Here's how the part is built. I have some questions about the finished solid (model axes, mm). Face numbers are marked on the shaded views. A direction names the side the tool comes from. Coordinates: 2 decimals unless noted, no trailing zeros. Write each loop counter-clockwise with the first axis right and the second up, starting at its lowest first coordinate (ties: lowest second). Pieces come first, ordered by that corner, then holes.
Item 1: I'm going to push flat-ended pins straight in: pin 1 Ø2 at (x, y) = (42.5, -18.5) entering from +Z (3 decimals); pin 2 Ø12 at (y, z) = (-23.5, 36) entering from +X; pin 3 Ø2 at (y, z) = (-110, 72.5) entering from +X. Where does each tip first touch, or does it pass through?
Item 2: If we section it at B-B (x = 30): Please give me the cut outline in (y, z) (3 decimals), then the cut area to 3 significant figures.
Item 3: We'd pull the mould along Z, two halves only. Please class the marked faces 1, 2 and 3: +Z half, -Z half, draft (parallel to the pull), parting line (faces both ways), or undercut.
Item 4: If we section it at A-A (z = 46): Please give me the cut outline in (x, y), then the cut area to 3 significant figures.
Item 5: For the marked faces 4 and 5, which set-ups out of +Z, -Z, +X, -X, +Y, -Y let a thin tool reach every point of the face, with its end or its side?
Item 6: If I drill on line 1 (Z direction, x = 29.5, y = -147) (3 decimals); line 2 (Z direction, x = 107.5, y = 131.5) (3 decimals); line 3 (Y direction, x = 68.5, z = 47), over which ranges is the centre line in solid material (lowest first)?
Item 7: If we section it at D-D (x = 147): Please give me the cut outline in (y, z) (3 decimals), then the cut area to 3 significant figures.
from build123d import *

# Parameters (mm, degrees)
F1_DEPTH = 3.175
F3_DEPTH = 76.2
F5_DEPTH = 3.175


with BuildPart() as f1:
    # F0 (on Top) → F1 (new body)
    with BuildSketch(Plane.XY):
        with BuildLine():
            ThreePointArc((0, 152.4), (23.5583821583, 150.5681328505), (46.5504148891, 145.1165699486))
            Line((46.5504148891, 145.1165699486), (76.2, 145.1165699486))
            Line((76.2, 145.1165699486), (76.2, 220.9699887776))
            Line((76.2, 220.9699887776), (0, 220.9699887776))
            Line((0, 220.9699887776), (0, 152.4))
        make_face()
        with BuildLine():
            Line((0, 145.1165699486), (46.5504148891, 145.1165699486))
            ThreePointArc((46.5504148891, 145.1165699486), (23.5583821583, 150.5681328505), (0, 152.4))
            Line((0, 152.4), (0, 145.1165699486))
        make_face()
        with BuildLine():
            Line((76.2, 79.9558987255), (76.2, 131.9822715367))
            ThreePointArc((76.2, 131.9822715367), (61.7255501195, 139.3402901621), (46.5504148891, 145.1165699486))
            Line((46.5504148891, 145.1165699486), (0, 145.1165699486))
            Line((0, 145.1165699486), (0, 102.5676841179))
            ThreePointArc((0, 102.5676841179), (39.7420836099, 96.795488514), (76.2, 79.9558987255))
        make_face()
        with BuildLine():
            Line((76.2, 30.069767419), (76.2, 79.9558987255))
            ThreePointArc((76.2, 79.9558987255), (39.7420836099, 96.795488514), (0, 102.5676841179))
            Line((0, 102.5676841179), (0, 64.4676841179))
            ThreePointArc((0, 64.4676841179), (41.802083301, 55.469767419), (76.2, 30.069767419))
        make_face()
        with BuildLine():
            ThreePointArc((134.4041666021, 0.9676841179), (112.4647200648, 45.7397345375), (76.2, 79.9558987255))
            Line((76.2, 79.9558987255), (76.2, 30.069767419))
            ThreePointArc((76.2, 30.069767419), (86.426594721, 16.2812004311), (94.1857207861, 0.9676841179))
            Line((94.1857207861, 0.9676841179), (134.4041666021, 0.9676841179))
        make_face()
        with BuildLine():
            ThreePointArc((94.1857207861, 0.9676841179), (86.426594721, 16.2812004311), (76.2, 30.069767419))
            Line((76.2, 30.069767419), (76.2, 0.9676841179))
            Line((76.2, 0.9676841179), (94.1857207861, 0.9676841179))
        make_face()
        with BuildLine():
            Line((94.1857207861, 0.9676841179), (76.2, 0.9676841179))
            Line((76.2, 0.9676841179), (76.2, -104.3343991831))
            ThreePointArc((76.2, -104.3343991831), (95.0380976241, -73.0533403663), (101.6, -37.1323158821))
            ThreePointArc((101.6, -37.1323158821), (99.7292064339, -17.7249620165), (94.1857207861, 0.9676841179))
        make_face()
        with BuildLine():
            ThreePointArc((0, -152.4), (39.4440224736, -147.2070959265), (76.2, -131.9822715367))
            Line((76.2, -131.9822715367), (76.2, -104.3343991831))
            ThreePointArc((76.2, -104.3343991831), (41.802083301, -129.7343991831), (0, -138.7323158821))
            Line((0, -138.7323158821), (0, -152.4))
        make_face()
        with BuildLine():
            Line((76.2, -104.3343991831), (76.2, 0.9676841179))
            Line((76.2, 0.9676841179), (0, 0.9676841179))
            Line((0, 0.9676841179), (0, -138.7323158821))
            ThreePointArc((0, -138.7323158821), (41.802083301, -129.7343991831), (76.2, -104.3343991831))
        make_face()
        with BuildLine():
            Line((76.2, -154.2205304897), (76.2, -131.9822715367))
            ThreePointArc((76.2, -131.9822715367), (39.4440224736, -147.2070959265), (0, -152.4))
            Line((0, -152.4), (0, -166.4440847683))
            Line((0, -166.4440847683), (52.8635642719, -166.4440847683))
            ThreePointArc((52.8635642719, -166.4440847683), (64.8205578921, -160.8836200148), (76.2, -154.2205304897))
        make_face()
        with BuildLine():
            Line((0, -236.2300112224), (76.2, -236.2300112224))
            Line((76.2, -236.2300112224), (76.2, -166.4440847683))
            Line((76.2, -166.4440847683), (52.8635642719, -166.4440847683))
            ThreePointArc((52.8635642719, -166.4440847683), (26.9372965106, -174.2106586525), (0, -176.8323158821))
            Line((0, -176.8323158821), (0, -236.2300112224))
        make_face()
        Polygon((76.2, -236.2300112224), (101.6, -166.4440847683), (76.2, -166.4440847683), align=None)
        with BuildLine():
            Line((76.2, -166.4440847683), (76.2, -154.2205304897))
            ThreePointArc((76.2, -154.2205304897), (64.8205578921, -160.8836200148), (52.8635642719, -166.4440847683))
            Line((52.8635642719, -166.4440847683), (76.2, -166.4440847683))
        make_face()
        with BuildLine():
            ThreePointArc((0, -176.8323158821), (26.9372965106, -174.2106586525), (52.8635642719, -166.4440847683))
            Line((52.8635642719, -166.4440847683), (0, -166.4440847683))
            Line((0, -166.4440847683), (0, -176.8323158821))
        make_face()
        with BuildLine():
            Line((101.6, -166.4440847683), (131.2750589092, -84.9125304942))
            ThreePointArc((131.2750589092, -84.9125304942), (109.372641612, -124.0444281957), (76.2, -154.2205304897))
            Line((76.2, -154.2205304897), (76.2, -166.4440847683))
            Line((76.2, -166.4440847683), (101.6, -166.4440847683))
        make_face()
        with BuildLine():
            ThreePointArc((131.2750589092, -84.9125304942), (133.9529126579, -76.7896883426), (136.1286754731, -68.5181998738))
            ThreePointArc((136.1286754731, -68.5181998738), (110.8051835658, -104.6325537056), (76.2, -131.9822715367))
            Line((76.2, -131.9822715367), (76.2, -154.2205304897))
            ThreePointArc((76.2, -154.2205304897), (109.372641612, -124.0444281957), (131.2750589092, -84.9125304942))
        make_face()
        with BuildLine():
            ThreePointArc((76.2, -131.9822715367), (110.8051835658, -104.6325537056), (136.1286754731, -68.5181998738))
            ThreePointArc((136.1286754731, -68.5181998738), (138.8042974183, -52.9265242574), (139.7, -37.1323158821))
            ThreePointArc((139.7, -37.1323158821), (138.3697078018, -17.8991683798), (134.4041666021, 0.9676841179))
            Line((134.4041666021, 0.9676841179), (94.1857207861, 0.9676841179))
            ThreePointArc((94.1857207861, 0.9676841179), (99.7292064339, -17.7249620165), (101.6, -37.1323158821))
            ThreePointArc((101.6, -37.1323158821), (95.0380976241, -73.0533403663), (76.2, -104.3343991831))
            Line((76.2, -104.3343991831), (76.2, -131.9822715367))
        make_face()
        with BuildLine():
            ThreePointArc((143.2091555839, -52.1238693589), (150.0847016038, -26.4639820229), (152.4, 0))
            ThreePointArc((152.4, 0), (131.9822715367, 76.2), (76.2, 131.9822715367))
            Line((76.2, 131.9822715367), (76.2, 79.9558987255))
            ThreePointArc((76.2, 79.9558987255), (112.4647200648, 45.7397345375), (134.4041666021, 0.9676841179))
            ThreePointArc((134.4041666021, 0.9676841179), (138.3697078018, -17.8991683798), (139.7, -37.1323158821))
            ThreePointArc((139.7, -37.1323158821), (138.8042974183, -52.9265242574), (136.1286754731, -68.5181998738))
            ThreePointArc((136.1286754731, -68.5181998738), (139.9092544586, -60.4248336103), (143.2091555839, -52.1238693589))
        make_face()
        with BuildLine():
            ThreePointArc((76.2, 131.9822715367), (131.9822715367, 76.2), (152.4, 0))
            ThreePointArc((152.4, 0), (150.0847016038, -26.4639820229), (143.2091555839, -52.1238693589))
            Line((143.2091555839, -52.1238693589), (242.6071911065, 220.9699887776))
            Line((242.6071911065, 220.9699887776), (76.2, 145.1165699486))
            Line((76.2, 145.1165699486), (76.2, 131.9822715367))
        make_face()
        with BuildLine():
            ThreePointArc((46.5504148891, 145.1165699486), (61.7255501195, 139.3402901621), (76.2, 131.9822715367))
            Line((76.2, 131.9822715367), (76.2, 145.1165699486))
            Line((76.2, 145.1165699486), (46.5504148891, 145.1165699486))
        make_face()
        Polygon((76.2, 220.9699887776), (76.2, 145.1165699486), (242.6071911065, 220.9699887776), align=None)
        with BuildLine():
            Line((131.2750589092, -84.9125304942), (143.2091555839, -52.1238693589))
            ThreePointArc((143.2091555839, -52.1238693589), (139.9092544586, -60.4248336103), (136.1286754731, -68.5181998738))
            ThreePointArc((136.1286754731, -68.5181998738), (133.9529126579, -76.7896883426), (131.2750589092, -84.9125304942))
        make_face()
    extrude(amount=F1_DEPTH)

    # F2 (on face) → F3 (join)
    with BuildSketch(Plane.XY.offset(3.175)):
        Polygon((242.6071911065, 220.9699887776), (239.2284266789, 220.9699887776), (73.9768410662, -233.0550112224), (77.3556054938, -233.0550112224), align=None)
        Polygon((77.3556054938, -233.0550112224), (73.9768410662, -233.0550112224), (72.8212355724, -236.2300112224), (76.2, -236.2300112224), align=None)
        Polygon((72.8212355724, -236.2300112224), (73.9768410662, -233.0550112224), (0, -233.0550112224), (0, -236.2300112224), align=None)
    extrude(amount=F3_DEPTH)

    # F4 (on face) → F5 (join)
    with BuildSketch(Plane.XY.offset(79.375)):
        Polygon((239.2284266789, 220.9699887776), (161.5176911065, 220.9699887776), (0, -222.7934112224), (0, -233.0550112224), (73.9768410662, -233.0550112224), align=None)
        Polygon((242.6071911065, 220.9699887776), (239.2284266789, 220.9699887776), (73.9768410662, -233.0550112224), (0, -233.0550112224), (0, -236.2300112224), (76.2, -236.2300112224), align=None)
    extrude(amount=F5_DEPTH)


solid = f1.part
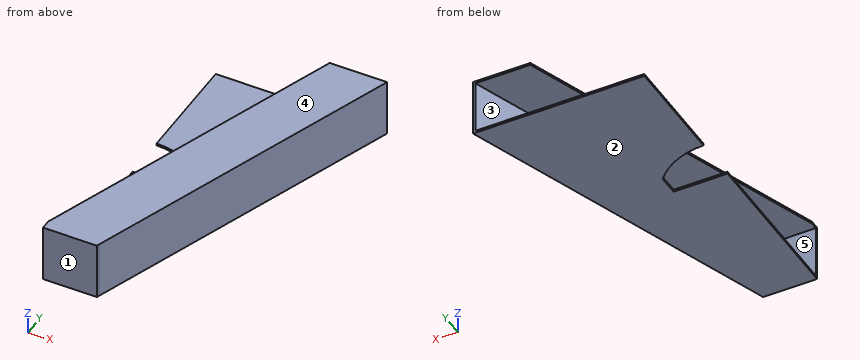
Answer list:
1. pin 1: stops at z = 3.175
1. pin 2: stops at x = 155.81
1. pin 3: stops at x = 122.51
2. outline: (-236.23, 0) - (0.968, 0) - (0.968, 3.175) - (-233.055, 3.175) - (-233.055, 79.375) - (-140.37, 79.375) - (-140.37, 82.55) - (-236.23, 82.55) - close; (59.938, 0) - (220.97, 0) - (220.97, 3.175) - (59.938, 3.175) - close
2. area: 1,810 mm2
3. face 1: draft
3. face 2: -Z half
3. face 3: undercut
4. outline: (0, -236.23) - (76.2, -236.23) - (242.61, 220.97) - (239.23, 220.97) - (73.98, -233.06) - (0, -233.06) - close
4. area: 1,780 mm2
5. face 4: +Z, +X, -X, +Y, -Y
5. face 5: -X, +Y
6. line 1: z = 0 to 3.175, 79.375 to 82.55
6. line 2: z = 0 to 3.175
6. line 3: y = -236.23 to -233.06
7. outline: (-41.709, 0) - (220.97, 0) - (220.97, 3.175) - (-32.426, 3.175) - (-32.426, 79.375) - (181.083, 79.375) - (181.083, 82.55) - (-41.709, 82.55) - close
7. area: 2,250 mm2
